Source: CAD feature listing. Evaluate the final solid. Frame: model axes, mm. Face numbers are marked on the shaded views. A direction names the side the tool comes from. Round coordinates to 2 decimals unless told otherwise and drop trailing zeros. Write each loop counter-clockwise with the first axis right and the second up, starting at its lowest first coordinate (ties: lowest second). Pieces come first, ordered by that corner, then holes. Notation, with made-up numbers: (-38.75, -27) - (18.25, -27) arc R13 ccw to (18.25, -5) - close; hole circle Ø9 at (79, 60). An arc over 180 degrees is marked (long way). Write item = value, one per line. Start each with the question number.
```python
from build123d import *

# Parameters (mm, degrees)
SKETCH_1_R          = 1.5
EXTRUDE_1_DEPTH     = 4
CUT_EXTRUDE_1_DEPTH = 3
FILLET_1_R          = 1


with BuildPart() as part:
    # 草图1 → 凸台-拉伸1 (new, symmetric)
    with BuildSketch(Plane(origin=(0, 0, 0), x_dir=(0, 0, -1), z_dir=(1, 0, 0))):
        with BuildLine():
            Line((0, 4), (18, 4))
            ThreePointArc((18, 4), (22, 0), (18, -4))
            Line((18, -4), (0, -4))
            ThreePointArc((0, -4), (-4, 0), (0, 4))
        make_face()
        Circle(SKETCH_1_R, mode=Mode.SUBTRACT)
        with Locations((18, 0)):
            Circle(SKETCH_1_R, mode=Mode.SUBTRACT)
    extrude(amount=EXTRUDE_1_DEPTH, both=True)

    # 草图2 → 切除-拉伸1 (cut)
    with BuildSketch(Plane(origin=(4, 0, 0), x_dir=(0, 0, -1), z_dir=(1, 0, 0))):
        with BuildLine():
            Line((3.122498999, -2.5), (14.877501001, -2.5))
            ThreePointArc((14.877501001, -2.5), (14, 0), (14.877501001, 2.5))
            Line((14.877501001, 2.5), (3.122498999, 2.5))
            ThreePointArc((3.122498999, 2.5), (4, 0), (3.122498999, -2.5))
        make_face()
    cut_extrude_1 = extrude(amount=-CUT_EXTRUDE_1_DEPTH, mode=Mode.SUBTRACT)

    # 镜向1: 切除-拉伸1 across plane
    add(cut_extrude_1.mirror(Plane(origin=(0, 0, 0), x_dir=(0, 0, 1), z_dir=(1, 0, 0))), mode=Mode.SUBTRACT)

    # 圆角1
    fillet_1_edges = [part.edges().sort_by_distance(p)[0] for p in [
        (2.5, 2.5, -14.877501001),
        (2.5, -2.5, -14.877501001),
        (2.5, -2.5, -3.122498999),
        (2.5, 2.5, -3.122498999),
        (-2.5, -2.5, -14.877501001),
        (-2.5, 2.5, -14.877501001),
        (-2.5, 2.5, -3.122498999),
        (-2.5, -2.5, -3.122498999),
    ]]
    fillet(fillet_1_edges, radius=FILLET_1_R)


solid = part.part
```
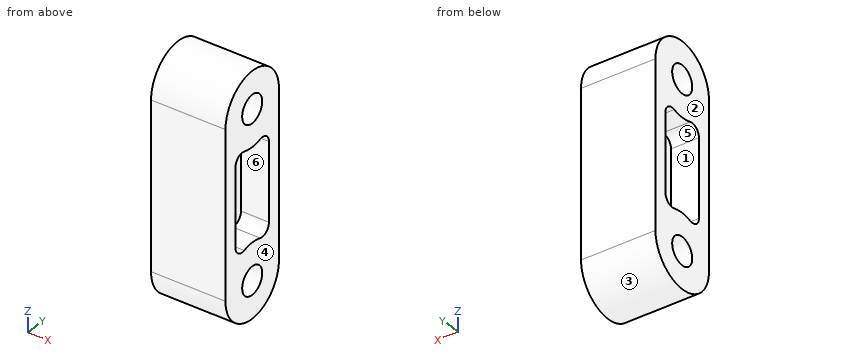
(1) Ray query, L1, parallel to Z at x = -0.25, y = -0.25; L2, parallel to Y at x = 0.75, z = -18; L3, parallel to Z at x = 2.75, y = -1.75. Return the intervals inside material, ascending. Write a range as from..to.
(2) Reachability of the marked faces 4, 5 and 6 from +Z, -Z, +X, -X, +Y, -Y: full face, straight path, thin tool, end or side. Return the list, or none.
(3) Section B-B (x = 2). Return the cut outline in (y, z).
(4) Pull-direction query (Y, two-part tool) for the marked faces 1, 2 and 3; classes: +Y half, -Y half, draft (parallel to the pull), parting line (faces both ways), or undercut.
(5) Contact query for flat-ended pins moving along their axis: P1, Ø2.5, axis at y = 0, z = -10, coming from the -X side; P2, Ø1, axis at x = -0.5, y = 1, coming from the -Z side; P3, Ø2, axis at x = 1, y = 2, coming from the -Z side. Output: stop coordinate, or through.
(6) Section D-D (x = 0). Return the cut outline in (y, z).
(7) Section A-A (y = 0). Return the cut outline in (x, z), plus the area to 3 significant figures.
(8) Section C-C (z = -9.25). Return the cut outline in (x, y), plus the area to 3 significant figures.
Solution:
q1.L1 = -21.99..-19.48, -16.52..-1.48, 1.48..3.99
q1.L2 = -4..-1.5, 1.5..4
q1.L3 = -21.6..-14.2, -3.8..3.6
q2.face_4 = +Z, -Z, +X, +Y, -Y
q2.face_5 = -X
q2.face_6 = +X
q3.outline = (-4, -18) arc R4 ccw to (4, -18) - (4, 0) arc R4 ccw to (-4, 0) - close; hole (-2.5, -13.23) arc R1 ccw to (-1.2, -14.18) arc R4 cw to (1.2, -14.18) arc R1 ccw to (2.5, -13.23) - (2.5, -4.77) arc R1 ccw to (1.2, -3.82) arc R4 cw to (-1.2, -3.82) arc R1 ccw to (-2.5, -4.77) - close; hole circle Ø3 at (0, -18); hole circle Ø3 at (0, 0)
q4.face_1 = undercut
q4.face_2 = draft
q4.face_3 = parting line
q5.P1 = -1
q5.P2 = -21.97
q5.P3 = -21.87
q6.outline = (-4, -18) arc R4 ccw to (4, -18) - (4, 0) arc R4 ccw to (-4, 0) - close; hole circle Ø3 at (0, -18); hole circle Ø3 at (0, 0)
q7.outline = (-4, -22) - (4, -22) - (4, -19.5) - (-4, -19.5) - close; (-4, -16.5) - (4, -16.5) - (4, -14) - (1, -14) - (1, -4) - (4, -4) - (4, -1.5) - (-4, -1.5) - (-4, -4) - (-1, -4) - (-1, -14) - (-4, -14) - close; (-4, 1.5) - (4, 1.5) - (4, 4) - (-4, 4) - close
q7.area = 100 mm^2
q8.outline = (-4, -4) - (4, -4) - (4, -2.5) - (1, -2.5) - (1, 2.5) - (4, 2.5) - (4, 4) - (-4, 4) - (-4, 2.5) - (-1, 2.5) - (-1, -2.5) - (-4, -2.5) - close
q8.area = 34.0 mm^2
